For this review, take the finished solid that the model builds, in its own axes (mm). A direction names the side the tool comes from. Give positions to 0.01 mm unless a question says otherwise; leave off trailing zeros. Write each loop counter-clockwise with the first axis right and the second up, starting at its lowest first coordinate (ties: lowest second). Pieces come first, ordered by that corner, then holes.
from build123d import *

# Parameters (mm, degrees)
SKETCH2_R          = 4.5
CUT_EXTRUDE1_DEPTH = 197.292186549
SKETCH4_R          = 4.4
CUT_EXTRUDE3_DEPTH = 18
SKETCH5_R          = 4.5
CUT_EXTRUDE4_DEPTH = 5
SKETCH6_R          = 1.5
CUT_EXTRUDE5_DEPTH = 8


with BuildPart() as part:
    # Sketch1 → Revolve1 (revolve)
    with BuildSketch(Plane(origin=(0, 0, 0), x_dir=(0, 0, -1), z_dir=(1, 0, 0)), mode=Mode.PRIVATE) as revolve1_sk:
        Polygon((-28, 0), (-35, 0), (-35, 34), (-39.3, 34), (-39.3, 44), (-84.5, 44), (-84.5, 55), (-95, 55), (-95.5, 57), (-97.5, 57), (-98, 55), (-111, 55), (-111, 117.85), (-88, 117.85), (-88, 122.85), (-46.5, 122.85), (-46.5, 113.65), (-28, 113.65), align=None)
    revolve(revolve1_sk.sketch.rotate(Axis((0, 0, 0), (0, 1, 0)), 180), axis=Axis((0, 0, 0), (0, 1, 0)))

    # Sketch2 → Cut-Extrude1 (cut, through all)
    with BuildSketch(Plane(origin=(0, 117.85, 0), x_dir=(1, 0, 0), z_dir=(0, 1, 0))):
        with Locations(Location((-104, 0, 0), (0, 0, 270))):
            Circle(SKETCH2_R)
        with Locations(Location((-73.539105243, 73.539105243, 0), (0, 0, 270))):
            Circle(SKETCH2_R)
        with Locations(Location((0, 104, 0), (0, 0, 270))):
            Circle(SKETCH2_R)
        with Locations(Location((73.539105243, 73.539105243, 0), (0, 0, 270))):
            Circle(SKETCH2_R)
        with Locations(Location((104, 0, 0), (0, 0, 270))):
            Circle(SKETCH2_R)
        with Locations(Location((73.539105243, -73.539105243, 0), (0, 0, 270))):
            Circle(SKETCH2_R)
        with Locations(Location((0, -104, 0), (0, 0, 270))):
            Circle(SKETCH2_R)
        with Locations(Location((-73.539105243, -73.539105243, 0), (0, 0, 270))):
            Circle(SKETCH2_R)
    extrude(amount=-CUT_EXTRUDE1_DEPTH, mode=Mode.SUBTRACT)

    # Sketch4 → Cut-Extrude3 (cut)
    with BuildSketch(Plane(origin=(0, 122.85, 0), x_dir=(1, 0, 0), z_dir=(0, 1, 0))):
        with Locations(Location((-66.5, 0, 0), (0, 0, 270))):
            Circle(SKETCH4_R)
        with Locations(Location((-61.437988912, 25.448448252, 0), (0, 0, 270))):
            Circle(SKETCH4_R)
        with Locations(Location((-25.448448252, 61.437988912, 0), (0, 0, 270))):
            Circle(SKETCH4_R)
        with Locations(Location((25.448448252, 61.437988912, 0), (0, 0, 270))):
            Circle(SKETCH4_R)
        with Locations(Location((61.437988912, 25.448448252, 0), (0, 0, 270))):
            Circle(SKETCH4_R)
        with Locations(Location((61.437988912, -25.448448252, 0), (0, 0, 270))):
            Circle(SKETCH4_R)
        with Locations(Location((25.448448252, -61.437988912, 0), (0, 0, 270))):
            Circle(SKETCH4_R)
        with Locations(Location((-25.448448252, -61.437988912, 0), (0, 0, 270))):
            Circle(SKETCH4_R)
        with Locations(Location((-61.437988912, -25.448448252, 0), (0, 0, 270))):
            Circle(SKETCH4_R)
    extrude(amount=-CUT_EXTRUDE3_DEPTH, mode=Mode.SUBTRACT)

    # Sketch5 → Cut-Extrude4 (cut)
    with BuildSketch(Plane(origin=(0, 122.85, 0), x_dir=(1, 0, 0), z_dir=(0, 1, 0))):
        with Locations(Location((0, -61.25, 0), (0, 0, 270))):
            Circle(SKETCH5_R)
        with Locations(Location((0, 61.25, 0), (0, 0, 270))):
            Circle(SKETCH5_R)
    extrude(amount=-CUT_EXTRUDE4_DEPTH, mode=Mode.SUBTRACT)

    # Sketch6 → Cut-Extrude5 (cut)
    with BuildSketch(Plane.XZ):
        with Locations(Location((0, 31.5, 0), (0, 0, 270))):
            Circle(SKETCH6_R)
        with Locations(Location((27.279800219, 15.75, 0), (0, 0, 270))):
            Circle(SKETCH6_R)
        with Locations(Location((27.279800219, -15.75, 0), (0, 0, 270))):
            Circle(SKETCH6_R)
        with Locations(Location((0, -31.5, 0), (0, 0, 270))):
            Circle(SKETCH6_R)
        with Locations(Location((-27.279800219, -15.75, 0), (0, 0, 270))):
            Circle(SKETCH6_R)
        with Locations(Location((-27.279800219, 15.75, 0), (0, 0, 270))):
            Circle(SKETCH6_R)
    extrude(amount=-CUT_EXTRUDE5_DEPTH, mode=Mode.SUBTRACT)


solid = part.part
(1) Clearance check with flat-ended pins moving along their axes: pin 1 Ø1.8 at (x, z) = (27.28, 15.75) entering from +Y; pin 2 Ø11.5 at (x, z) = (-25.45, 61.44) entering from -Y; pin 3 Ø3 at (y, z) = (64, -23.5) entering from -X. State where each tip first meets the part, or that it passes through.
(2) For L1, parallel to X at y = 105, z = 0; L2, parallel to X at y = 105.5, z = -70; L3, parallel to X at y = 52, z = 0.5, list the stretches that pass through material, from the lowest coordinate up.
(3) We need section B-B (x = -104). Write out the cut boundary in (y, z).
(4) The part is to be moulded in two halves that separate along Z. For faces 4 (the flat face through (38, 122.85, -38)), 5 (the cylindrical face through (-38.966, 39.07, 5.116)), 6 (the cylindrical face through (0.198, 86.865, -108.496)), 7 (the flat face through (-61, 104.85, 25)), say which applies: +Z half, -Z half, draft (parallel to the pull), parting line (faces both ways), or undercut.
(5) We need section A-A (z = 104). Write out the cut boundary in (x, y).
(6) Tool access review of faces 1 (the flat face through (98.15, 55, -0.52)), 2 (the cylindrical face through (69.55, 86.86, -71.46)), 3 (the flat face through (20, 113.65, -20)): name each direction out of +Z, -Z, +X, -X, +Y, -Y from which nothing blocks a thin tool from reaching the whole face with its end or side.
(7) We need section D-D (y = 73.5). Count the separate pieces of the cut face and the enclosed holes in it, and give its area (3 significant figures).
(8) We need section C-C (y = 19). Write out the cut boundary in (x, z), and give its area (3 significant figures).
The answers:
1. pin 1: stops at y = 113.65
1. pin 2: stops at y = 44
1. pin 3: stops at x = -108.8
2. L1: x = -111 to -108.5, -99.5 to -70.9, -62.1 to -28, 28 to 99.5, 108.5 to 111
2. L2: x = -86.15 to -76.32, -70.76 to 70.76, 76.32 to 86.15
2. L3: x = -84.5 to -28, 28 to 84.5
3. outline: (55, -38.79) - (117.85, -38.79) - (117.85, -4.5) - (55, -4.5) - close; (55, 4.5) - (117.85, 4.5) - (117.85, 38.79) - (55, 38.79) - close
4. face 4: draft
4. face 5: parting line
4. face 6: undercut
4. face 7: undercut
5. outline: (-38.79, 55) - (-4.5, 55) - (-4.5, 117.85) - (-38.79, 117.85) - close; (4.5, 55) - (38.79, 55) - (38.79, 117.85) - (4.5, 117.85) - close
6. face 1: -Y
6. face 2: +Y, -Y
6. face 3: +Y
7. separate pieces: 1
7. enclosed holes: 9
7. area: 35,700 mm2
8. outline: circle Ø70 at (0, 0); hole circle Ø56 at (0, 0)
8. area: 1,390 mm2
